Read the model definition and answer for the solid it produces. Units are mm, in the model's axes. Give positions to 0.01 mm unless a question says otherwise; leave off trailing zeros. Order: outer loops, then holes, each group sorted by start corner. A loop starts at its lowest first (then second) coordinate and runs counter-clockwise, first axis right, second up. Notation, with made-up numbers: (57, 1.25) -> (113, 1.25) arc R11 ccw to (113, 12.25) -> close; hole circle Ø6 at (-8.5, 31.5). An arc over 180 degrees is marked (long way). One line per question, with ' | ' between items. Start each with the question number.
```python
from build123d import *

# Parameters (mm, degrees)
SKETCH_1_W          = 91
SKETCH_1_H          = 42
EXTRUDE_1_DEPTH     = 5
SKETCH_2_R          = 1.75
SKETCH_2_R_2        = 2.25
SKETCH_2_R_3        = 1.9
CUT_EXTRUDE_1_DEPTH = 5
SKETCH_3_R          = 4
SKETCH_3_R_2        = 3.25
CUT_EXTRUDE_2_DEPTH = 5


with BuildPart() as part:
    # 스케치1 → 보스-돌출1 (new body)
    with BuildSketch(Plane(origin=(0, 0, 0), x_dir=(1, 0, 0), z_dir=(0, 1, 0))):
        with Locations((45.5, 21)):
            Rectangle(SKETCH_1_W, SKETCH_1_H)
    extrude(amount=EXTRUDE_1_DEPTH)

    # 스케치2 → 컷-돌출1 (cut)
    with BuildSketch(Plane(origin=(0, 5, 0), x_dir=(1, 0, 0), z_dir=(0, 1, 0))):
        with Locations(Location((28, 33.5, 0), (0, 0, 270))):
            Circle(SKETCH_2_R)
        with Locations(Location((28, 8.5, 0), (0, 0, 270))):
            Circle(SKETCH_2_R)
        with Locations(Location((8, 8.5, 0), (0, 0, 270))):
            Circle(SKETCH_2_R)
        with Locations(Location((8, 33.5, 0), (0, 0, 270))):
            Circle(SKETCH_2_R)
        with Locations(Location((42.094873015, 28, 0), (0, 0, 270))):
            Circle(SKETCH_2_R_2)
        with Locations(Location((42.094873015, 14, 0), (0, 0, 270))):
            Circle(SKETCH_2_R_2)
        with Locations(Location((84.094873015, 14, 0), (0, 0, 270))):
            Circle(SKETCH_2_R_2)
        with Locations(Location((84.094873015, 28, 0), (0, 0, 270))):
            Circle(SKETCH_2_R_2)
        with Locations(Location((78, 21, 0), (0, 0, 270))):
            Circle(SKETCH_2_R_3)
        with Locations(Location((13, 21, 0), (0, 0, 270))):
            Circle(SKETCH_2_R_3)
    extrude(amount=-CUT_EXTRUDE_1_DEPTH, mode=Mode.SUBTRACT)

    # 스케치3 → 컷-돌출2 (cut)
    with BuildSketch(Plane(origin=(0, 5, 0), x_dir=(1, 0, 0), z_dir=(0, 1, 0))):
        with Locations(Location((84.094873015, 28, 0), (0, 0, 270))):
            Circle(SKETCH_3_R)
        with Locations(Location((84.094873015, 14, 0), (0, 0, 270))):
            Circle(SKETCH_3_R)
        with Locations(Location((42.094873015, 14, 0), (0, 0, 270))):
            Circle(SKETCH_3_R)
        with Locations(Location((42.094873015, 28, 0), (0, 0, 270))):
            Circle(SKETCH_3_R)
        with Locations(Location((28, 33.5, 0), (0, 0, 270))):
            Circle(SKETCH_3_R_2)
        with Locations(Location((28, 8.5, 0), (0, 0, 270))):
            Circle(SKETCH_3_R_2)
        with Locations(Location((8, 8.5, 0), (0, 0, 270))):
            Circle(SKETCH_3_R_2)
        with Locations(Location((8, 33.5, 0), (0, 0, 270))):
            Circle(SKETCH_3_R_2)
    extrude(amount=-CUT_EXTRUDE_2_DEPTH, mode=Mode.SUBTRACT)


solid = part.part
```
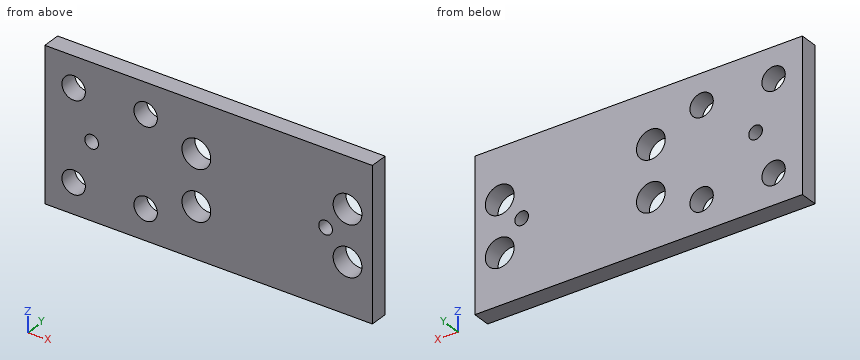
Q1. Find the intervals of material crossed by line 1 (X direction, y = 2.3, z = -8.5); line 2 (X direction, y = 1.95, z = -28); line 3 (Z direction, x = 82, y = 1.05), in increasing order.
Q2. A cutting plane is placed at B-B, the plane z = -33.5. Determine the outline of the cut face in (x, y), then the cut area to 3 significant figures.
Q3. A cutting plane is placed at A-A, the plane x = 28. Determine the outline of the cut face in (y, z), then the cut area to 3 significant figures.
Q4. A cutting plane is placed at C-C, the plane y = 1.65. Give the number of separate pieces and of enclosed holes in the cut face, then the cut area to 3 significant figures.
Q5. A cutting plane is placed at D-D, the plane x = 77. Determine the outline of the cut face in (y, z).
Geometry results:
1) line 1: 0 to 4.75, 11.25 to 24.75, 31.25 to 91 | line 2: 0 to 38.09, 46.09 to 80.09, 88.09 to 91 | line 3: -42 to -31.41, -24.59 to -17.41, -10.59 to 0
2) outline: (0, 0) -> (4.75, 0) -> (4.75, 5) -> (0, 5) -> close; (11.25, 0) -> (24.75, 0) -> (24.75, 5) -> (11.25, 5) -> close; (31.25, 0) -> (91, 0) -> (91, 5) -> (31.25, 5) -> close | area: 390 mm²
3) outline: (0, -42) -> (5, -42) -> (5, -36.75) -> (0, -36.75) -> close; (0, -30.25) -> (5, -30.25) -> (5, -11.75) -> (0, -11.75) -> close; (0, -5.25) -> (5, -5.25) -> (5, 0) -> (0, 0) -> close | area: 145 mm²
4) separate pieces: 1 | enclosed holes: 10 | area: 3,470 mm²
5) outline: (0, -42) -> (5, -42) -> (5, -22.62) -> (0, -22.62) -> close; (0, -19.38) -> (5, -19.38) -> (5, 0) -> (0, 0) -> close
